Check sheet for the modelled part. Datum: model origin and axes. Units: mm. A direction names the side the tool comes from. Coordinates: 2 decimals unless noted, no trailing zeros. Loops run counter-clockwise (first coordinate to the right, second up) from the corner with the lowest first, then second, coordinate; pieces in that order, holes last.
```python
from build123d import *

# Parameters (mm, degrees)
F0_R      = 63.5
F1_DEPTH  = 25.4
F2_R      = 66.675
F2_R_2    = 60.325
F3_DEPTH  = 25.4
F4_R      = 73.025
F4_R_2    = 63.5
F5_DEPTH  = 25.4
F6_R      = 66.675
F6_R_2    = 57.15
F7_DEPTH  = 25.4
F8_R      = 60.325
F8_R_2    = 49.53
F9_DEPTH  = 25.4
F10_R     = 54.61
F11_DEPTH = 25.4
F13_D     = 17.78
F13_DEPTH = 73.026


with BuildPart() as f1:
    # F0 (on Front) → F1 (new body)
    with BuildSketch(Plane.XZ):
        Circle(F0_R)
    extrude(amount=F1_DEPTH)

    # F2 (on face) → F3 (join)
    with BuildSketch(Plane(origin=(0, 0, 0), x_dir=(-1, 0, 0), z_dir=(0, 1, 0))):
        Circle(F2_R)
        Circle(F2_R_2, mode=Mode.SUBTRACT)
    extrude(amount=F3_DEPTH)

    # F4 (on face) → F5 (join)
    with BuildSketch(Plane(origin=(0, 25.4, 0), x_dir=(-1, 0, 0), z_dir=(0, 1, 0))):
        Circle(F4_R)
        Circle(F4_R_2, mode=Mode.SUBTRACT)
    extrude(amount=F5_DEPTH)

    # F6 (on face) → F7 (join)
    with BuildSketch(Plane(origin=(0, 50.8, 0), x_dir=(-1, 0, 0), z_dir=(0, 1, 0))):
        Circle(F6_R)
        Circle(F6_R_2, mode=Mode.SUBTRACT)
    extrude(amount=F7_DEPTH)

    # F8 (on face) → F9 (join)
    with BuildSketch(Plane(origin=(0, 76.2, 0), x_dir=(-1, 0, 0), z_dir=(0, 1, 0))):
        Circle(F8_R)
        Circle(F8_R_2, mode=Mode.SUBTRACT)
    extrude(amount=F9_DEPTH)

    # F10 (on face) → F11 (join)
    with BuildSketch(Plane(origin=(0, 101.6, 0), x_dir=(-1, 0, 0), z_dir=(0, 1, 0))):
        Circle(F10_R)
    extrude(amount=F11_DEPTH)

    # F13 (through all, one way)
    with BuildSketch(Plane(origin=(0, 0, 0), x_dir=(1, 0, 0), z_dir=(0, 0, -1))):
        with Locations((-27.1317604929, -37.2066497803)):
            Circle(F13_D / 2)
    extrude(amount=-F13_DEPTH, mode=Mode.SUBTRACT)


solid = f1.part
```
1) Section check C-C on y = 73.5. Enter the section's corners in (x, z) (3 decimals), plus the area to 3 significant figures.
Answer sheet:
outline: circle Ø133.35 at (0, 0); hole circle Ø114.3 at (0, 0)
area: 3,710 mm2
2) Mould release check, pull along X, two halves, no side actions. Record for faces 1 (the cylindrical face through (60.267, 88.722, 2.652)), 2 (the flat face through (-59, 0, -24)), 3 (the cylindrical face through (57.095, 63.322, 2.513)): +X half, -X half, draft (parallel to the pull), parting line (faces both ways), or undercut.
Answer sheet:
face 1: parting line
face 2: draft
face 3: undercut
3) Section check A-A on y = 9.5. Enter the section's corners in (x, z) (3 decimals), plus the area to 3 significant figures.
Answer sheet:
outline: circle Ø133.35 at (0, 0); hole circle Ø120.65 at (0, 0)
area: 2,530 mm2
4) Set-up check for faces 4 (the cylindrical face through (-47.24, 88.72, 14.88)), 5 (the flat face through (-32, 25.4, -59)), 6 (the flat face through (15, 76.2, -59)), 7 (the cylindrical face through (-34.2, 42.6, 61.4)): record each of +Z, -Z, +X, -X, +Y, -Y from which the full face is reachable in a straight line by a thin tool's end or side.
Answer sheet:
face 4: none
face 5: -Y
face 6: +Y
face 7: +Z
5) Section check B-B on y = -15. Enter the section's corners in (x, z).
Answer sheet:
outline: circle Ø127 at (0, 0)
6) Depth check by flat-ended pin: pin 1 (1 mm diameter, centred on y = 18, z = -4, fed in from +X); pin 2 (2 mm diameter, centred on y = 22.5, z = 32, fed in from -X); pin 3 (8 mm diameter, centred on x = 12.5, y = 13.5, fed in from -Z). Enter the tip coordinate at first touch or a pass-through.
Answer sheet:
pin 1: stops at x = 66.58
pin 2: stops at x = -59.03
pin 3: stops at z = -66.13
7) Scan lines: line 1 (Z direction, x = 0, y = 83) (3 decimals); line 2 (Y direction, x = 0, z = -1); line 3 (Y direction, x = 7, z = -61). Record each from-to range of solid material in increasing order.
Answer sheet:
line 1: z = -60.325 to -49.53, 49.53 to 60.325
line 2: y = -25.4 to 0, 101.6 to 127
line 3: y = -25.4 to 25.4, 50.8 to 76.2
